```python
from build123d import *

# Parameters (mm, degrees)
F1_DEPTH = 38.1
F2_T     = -2.54
F3_W     = 7.62
F3_H     = 15.24
F4_DEPTH = 19.05
F5_R     = 5.08
F6_R     = 4.594696
F7_DEPTH = 39.878


with BuildPart() as f1:
    # F0 (on Right) → F1 (new body, symmetric)
    with BuildSketch(Plane.YZ):
        Polygon((37.679132, -31.786919), (37.679132, 21.553082), (-8.528198, -31.786919), align=None)
    extrude(amount=F1_DEPTH, both=True)

    # F2
    f2_openings = [f1.faces().sort_by_distance(p)[0] for p in [
        (0, 14.575467, -5.116918),
    ]]
    offset(amount=F2_T, openings=f2_openings)

    # F3 (on face) → F4 (join)
    with BuildSketch(Plane(origin=(0, 37.679132, 0), x_dir=(-1, 0, 0), z_dir=(0, 1, 0))):
        with Locations((-12.7, 0)):
            Rectangle(F3_W, F3_H)
        with Locations((12.7, 0)):
            Rectangle(F3_W, F3_H)
    extrude(amount=F4_DEPTH)

    # F5
    f5_edges = [f1.edges().sort_by_distance(p)[0] for p in [
        (12.7, 56.729132, 7.62),
        (12.7, 56.729132, -7.62),
        (-12.7, 56.729132, -7.62),
        (-12.7, 56.729132, 7.62),
    ]]
    fillet(f5_edges, radius=F5_R)

    # F6 (on face) → F7 (cut)
    with BuildSketch(Plane(origin=(-16.51, 0, 0), x_dir=(0, -1, 0), z_dir=(-1, 0, 0))):
        with Locations((-47.819119, 0)):
            Circle(F6_R)
    extrude(amount=-F7_DEPTH, mode=Mode.SUBTRACT)


solid = f1.part
```
Part model, mm, in its own coordinate system. A direction names the side the tool comes from. Give positions to 0.01 mm unless a question says otherwise; leave off trailing zeros. Order: outer loops, then holes, each group sorted by start corner. A loop starts at its lowest first (then second) coordinate and runs counter-clockwise, first axis right, second up. Notation, with made-up numbers: (-13.75, 75) - (-6.75, 75) arc R11 ccw to (-6.75, 89) - close; hole circle Ø6 at (37.25, 27.5). An arc over 180 degrees is marked (long way). Use one line per item in the form item = value.
Item 1: Slice it at D-D on z = 6. Give the cut face in (x, y), and give its area (3 significant figures).
Solution:
outline = (-38.1, 24.21) - (-35.56, 24.21) - (-35.56, 35.14) - (35.56, 35.14) - (35.56, 24.21) - (38.1, 24.21) - (38.1, 37.68) - (16.51, 37.68) - (16.51, 55.37) - (8.89, 55.37) - (8.89, 37.68) - (-8.89, 37.68) - (-8.89, 55.37) - (-16.51, 55.37) - (-16.51, 37.68) - (-38.1, 37.68) - close
area = 519 mm2
Item 2: Slice it at A-A on y = 41.5. Give the cut face in (x, z), and give its area (3 significant figures).
Solution:
outline = (-16.51, -7.62) - (-8.89, -7.62) - (-8.89, 7.62) - (-16.51, 7.62) - close; (8.89, -7.62) - (16.51, -7.62) - (16.51, 7.62) - (8.89, 7.62) - close
area = 232 mm2
Item 3: Pin check, flat tips, straight feed: pin 1 Ø20.5 at (y, z) = (7.5, -4) entering from +X; pin 2 Ø8 at (x, z) = (4.5, -19) entering from +Y; pin 3 Ø17 at (y, z) = (51.5, -3) entering from -X; pin 4 Ø4 at (x, y) = (12, 46) entering from -Z. Stop position of each tip, or through.
Solution:
pin_1 = 38.1
pin_2 = 37.68
pin_3 = -16.51
pin_4 = -7.62
Item 4: Slice it at B-B on x = 32. Give the cut face in (y, z).
Solution:
outline = (-8.53, -31.79) - (37.68, -31.79) - (37.68, 21.55) - (35.14, 18.62) - (35.14, -29.25) - (-6.33, -29.25) - close
Item 5: Two-plate mould, pull along Y, no slides. Class faces 1 (the face through (-12.753, 55.202, -6.171)), 2 (the face through (12.65, 52.41, 0.2)), 3 (the face through (-2.64, 36.93, 20.69)), 4 (the face through (1, 14, -31.787)): released by +Y, released by -Y, zero draft, split by the parting line, or undercut.
Solution:
face_1 = released by +Y
face_2 = undercut
face_3 = released by -Y
face_4 = zero draft
Item 6: Which spindle directions (+Z, -Z, +X, -X, +Y, -Y) get a long thin tool onto all of the face, cutting with end or side? Do faces 5 (the face through (13, 45, 7.62)), 6 (the face through (-35.56, 23, -16)), 7 (the face through (16.51, 43, 0)). Say none if no direction does.
Solution:
face_5 = +Z, +X, -X, +Y
face_6 = +Z, -Y
face_7 = +Z, -Z, +X, +Y
Item 7: Slice it at C-C on z = 0. Give the cut face in (x, y).
Solution:
outline = (-38.1, 19.01) - (-35.56, 19.01) - (-35.56, 35.14) - (35.56, 35.14) - (35.56, 19.01) - (38.1, 19.01) - (38.1, 37.68) - (16.51, 37.68) - (16.51, 43.22) - (8.89, 43.22) - (8.89, 37.68) - (-8.89, 37.68) - (-8.89, 43.22) - (-16.51, 43.22) - (-16.51, 37.68) - (-38.1, 37.68) - close; (-16.51, 52.41) - (-8.89, 52.41) - (-8.89, 56.73) - (-16.51, 56.73) - close; (8.89, 52.41) - (16.51, 52.41) - (16.51, 56.73) - (8.89, 56.73) - close
Item 8: Probe probe 1 along X at (y, z) = (4, -25.5); probe 2 along Y at (x, z) = (5.5, -1.5); probe 3 along Z at (x, y) = (-11, 8.5). List the from-to ranges inside material, lowest first. Write a range as from..to.
Solution:
probe_1 = -38.1..-35.56, 35.56..38.1
probe_2 = 35.14..37.68
probe_3 = -31.79..-29.25
